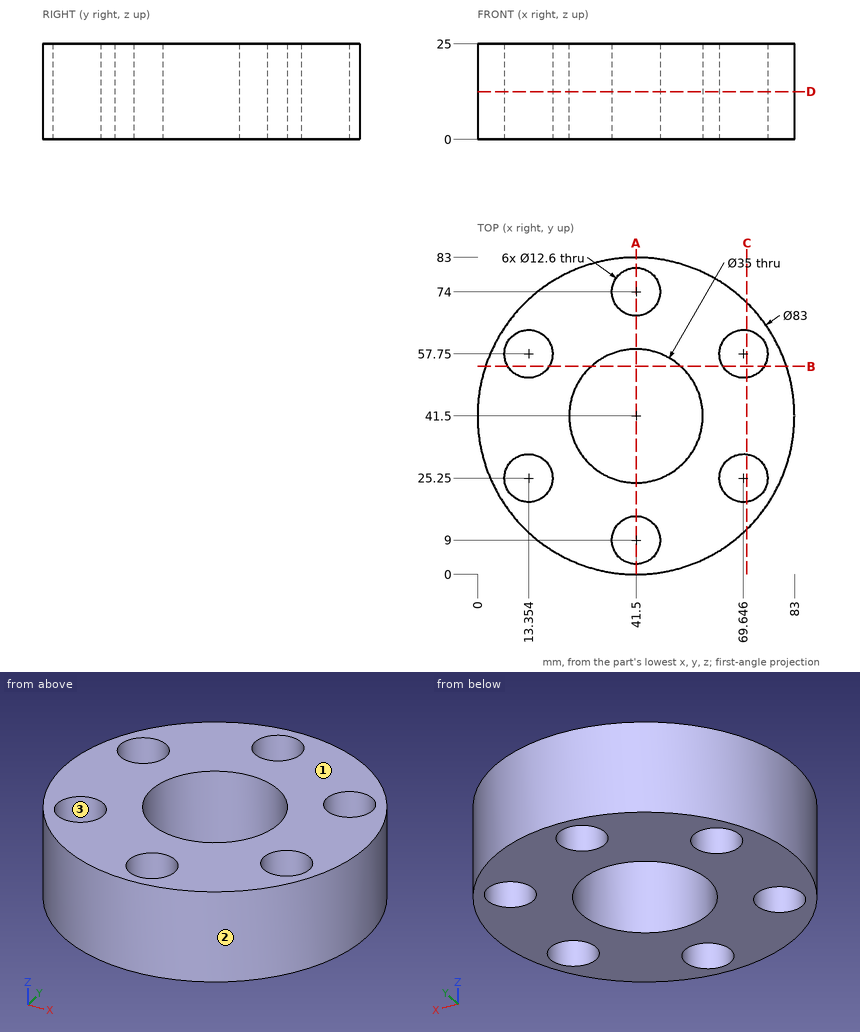
Study the drawing (mm; zero at the part's minimum x, y, z) and answer. Give positions to 0.01 mm unless a question says otherwise; leave off trailing zeros. Write each loop counter-clockwise with the first axis right and the second up, starting at its lowest first coordinate (ties: lowest second). Pieces come first, ordered by that corner, then holes.
(1) The part is cut by section C-C on x = 70.5. Write down the section's boundary in (y, z).
Final values:
outline: (11.81, 0) - (19.01, 0) - (19.01, 25) - (11.81, 25) - close; (31.49, 0) - (51.51, 0) - (51.51, 25) - (31.49, 25) - close; (63.99, 0) - (71.19, 0) - (71.19, 25) - (63.99, 25) - close
(2) The part is cut by section B-B on y = 54.5. Write down the section's boundary in (x, z), plus the area to 3 significant figures.
Final values:
outline: (2.09, 0) - (7.96, 0) - (7.96, 25) - (2.09, 25) - close; (18.75, 0) - (29.78, 0) - (29.78, 25) - (18.75, 25) - close; (53.22, 0) - (64.25, 0) - (64.25, 25) - (53.22, 25) - close; (75.04, 0) - (80.91, 0) - (80.91, 25) - (75.04, 25) - close
area: 845 mm2
(3) The mould has two halves that part along Y. Classify the marked faces 1, 2 and 3: pulls with the +Y half, pulls with the -Y half, needs draft (parallel to the pull), parting line crosses it, or undercut.
Final values:
face 1: needs draft
face 2: parting line crosses it
face 3: undercut
(4) The part is cut by section A-A on x = 41.5. Write down the section's boundary in (y, z).
Final values:
outline: (0, 0) - (2.7, 0) - (2.7, 25) - (0, 25) - close; (15.3, 0) - (24, 0) - (24, 25) - (15.3, 25) - close; (59, 0) - (67.7, 0) - (67.7, 25) - (59, 25) - close; (80.3, 0) - (83, 0) - (83, 25) - (80.3, 25) - close
(5) Flat-ended cylindrical pins translate along their axes: pin 1 Ø14.5 at (x, y) = (41.5, 9) entering from -Z; pin 2 Ø2 at (x, z) = (74, 13.5) entering from +Y; pin 3 Ø10 at (x, z) = (47, 12.5) entering from +Y; pin 4 Ø4 at (x, z) = (53.5, 22.5) entering from -Y. Find the tip coordinate at first contact, or state that the pin passes through.
Final values:
pin 1: stops at z = 0
pin 2: stops at y = 68.52
pin 3: stops at y = 83
pin 4: stops at y = 1.22
(6) Straight lines are drawn through the part: line 1 (Y direction, x = 41.5, z = 18.25); line 2 (Y direction, x = 9, z = 14.25); line 3 (Y direction, x = 10, z = 18.25). For each, find the intervals that lie inside material, in ascending order.
Final values:
line 1: y = 0 to 2.7, 15.3 to 24, 59 to 67.7, 80.3 to 83
line 2: y = 15.69 to 20.7, 29.8 to 53.2, 62.3 to 67.31
line 3: y = 14.48 to 19.92, 30.58 to 52.42, 63.08 to 68.52
(7) The part is cut by section D-D on z = 12.5. Write down the section's boundary in (x, y).
Final values:
outline: circle Ø83 at (41.5, 41.5); hole circle Ø12.6 at (13.35, 25.25); hole circle Ø12.6 at (13.35, 57.75); hole circle Ø35 at (41.5, 41.5); hole circle Ø12.6 at (41.5, 9); hole circle Ø12.6 at (41.5, 74); hole circle Ø12.6 at (69.65, 25.25); hole circle Ø12.6 at (69.65, 57.75)
